Model file for the job. Use its own axes, mm. A direction names the side the tool comes from. Round coordinates to 2 decimals unless told otherwise and drop trailing zeros. Order: outer loops, then holes, each group sorted by start corner. A loop starts at its lowest first (then second) coordinate and runs counter-clockwise, first axis right, second up. Notation, with made-up numbers: (21, 48) - (29, 48) arc R29 ccw to (29, 76) - close; hole circle Ø9 at (62, 1.5). An arc over 180 degrees is marked (long way). Put each result on its own line as item: value. Start each with the question number.
Item 1: Mould opens along Y. For faces 5 (the face through (-33, 42.5, 49)), 6 (the face through (-33.45, -34.95, 14.95)), 7 (the face through (-37, 1, 49)) say: pulls with the +Y half, pulls with the -Y half, needs draft (parallel to the pull), parting line crosses it, or undercut.
Item 2: Which spindle directions (+Z, -Z, +X, -X, +Y, -Y) get a long thin tool onto all of the face, cutting with end or side? Do faces 1 (the face through (-7.378, 10.417, 3.549)), 2 (the face through (-15, -22.5, 49)), 3 (the face through (-30, 32, 49)), 4 (the face through (-20.274, 0.057, 54.151)). Say none if no direction does.
Item 3: Saw through at A-A on z = 38.1. List the corners of the cut face in (x, y) (3 decimals).
Item 4: Pin check, flat tips, straight feed: pin 1 Ø24 at (x, z) = (-10.5, 39) entering from +Y; pin 2 Ø8.5 at (y, z) = (32.5, 63.5) entering from +X; pin 3 Ø5 at (x, z) = (10.5, 28.5) entering from -Y; pin 4 Ø3 at (x, y) = (-7, -12.13) entering from -Z. Stop position of each tip, or through.
Item 5: Saw through at C-C on x = 14. List the corners of the cut face in (y, z), plus the area to 3 significant figures.
Item 6: Probe probe 1 along Z at (x, y) = (-34.75, 32.5) (3 decimals); probe 2 along Y at (x, z) = (-32, 63); probe 3 along Y at (x, z) = (-29.5, 17.5). List the from-to ranges inside material, lowest first.
Item 7: Saw through at D-D on y = 4. List the corners of the cut face in (x, z).
Item 8: Saw through at B-B on y = -32.5. List the corners of the cut face in (x, z) (3 decimals), plus the area to 3 significant figures.
```python
from build123d import *

# Parameters (mm, degrees)
F1_DEPTH = 100
F3_DEPTH = 93
F4_R     = 10.75
F4_R_2   = 1.75
F5_DEPTH = 7.001
F6_R     = 3.325
F7_DEPTH = 7.001


with BuildPart() as f1:
    # F0 (on Top) → F1 (new body)
    with BuildSketch(Plane.XY):
        with BuildLine():
            Line((-30, -22.5), (0, -22.5))
            ThreePointArc((0, -22.5), (22.5, 0), (0, 22.5))
            Line((0, 22.5), (-30, 22.5))
            Line((-30, 22.5), (-30, 42.5))
            Line((-30, 42.5), (-37, 42.5))
            Line((-37, 42.5), (-37, -42.5))
            Line((-37, -42.5), (-30, -42.5))
            Line((-30, -42.5), (-30, -22.5))
        make_face()
    extrude(amount=F1_DEPTH)

    # F2 (on face) → F3 (cut)
    with BuildSketch(Plane.XY.offset(100)):
        with BuildLine():
            ThreePointArc((10.9589791569, -13.9946918808), (15.9804017395, -7.7831475152), (17.775, 0))
            ThreePointArc((17.775, 0), (15.9804017395, 7.7831475152), (10.9589791569, 13.9946918808))
            ThreePointArc((10.9589791569, 13.9946918808), (7.6371976915, 13.2287125761), (6.6395155094, 16.4884037675))
            ThreePointArc((6.6395155094, 16.4884037675), (-8.8876758914, 15.3935), (-17.5991912799, 2.493810597))
            ThreePointArc((-17.5991912799, 2.493810597), (-15.9461312513, 1.7044761952), (-15.275, 0))
            ThreePointArc((-15.275, 0), (-15.9461312513, -1.7044761952), (-17.5991912799, -2.493810597))
            ThreePointArc((-17.5991912799, -2.493810597), (-8.8876758914, -15.3935), (6.6395155094, -16.4884037675))
            ThreePointArc((6.6395155094, -16.4884037675), (7.6371976915, -13.2287125761), (10.9589791569, -13.9946918808))
        make_face()
        with BuildLine():
            ThreePointArc((6.6395155094, 16.4884037675), (7.6371976915, 13.2287125761), (10.9589791569, 13.9946918808))
            ThreePointArc((10.9589791569, 13.9946918808), (8.8871482138, 15.3938046508), (6.6395155094, 16.4884037675))
        make_face()
        with BuildLine():
            ThreePointArc((6.6395155094, 16.4884037675), (8.8871482138, 15.3938046508), (10.9589791569, 13.9946918808))
            ThreePointArc((10.9589791569, 13.9946918808), (11.2777106327, 14.662223267), (11.3871482138, 15.3938046508))
            ThreePointArc((11.3871482138, 15.3938046508), (9.4488056891, 17.8298959628), (6.6395155094, 16.4884037675))
        make_face()
        with BuildLine():
            ThreePointArc((11.3871482138, -15.3938046508), (11.2777106327, -14.662223267), (10.9589791569, -13.9946918808))
            ThreePointArc((10.9589791569, -13.9946918808), (8.8871482138, -15.3938046508), (6.6395155094, -16.4884037675))
            ThreePointArc((6.6395155094, -16.4884037675), (9.4488056891, -17.8298959628), (11.3871482138, -15.3938046508))
        make_face()
        with BuildLine():
            ThreePointArc((6.6395155094, -16.4884037675), (8.8871482138, -15.3938046508), (10.9589791569, -13.9946918808))
            ThreePointArc((10.9589791569, -13.9946918808), (7.6371976915, -13.2287125761), (6.6395155094, -16.4884037675))
        make_face()
        with BuildLine():
            ThreePointArc((-15.275, 0), (-15.9461312513, 1.7044761952), (-17.5991912799, 2.493810597))
            ThreePointArc((-17.5991912799, 2.493810597), (-17.775, 0), (-17.5991912799, -2.493810597))
            ThreePointArc((-17.5991912799, -2.493810597), (-15.9461312513, -1.7044761952), (-15.275, 0))
        make_face()
        with BuildLine():
            ThreePointArc((-17.5991912799, -2.493810597), (-17.775, 0), (-17.5991912799, 2.493810597))
            ThreePointArc((-17.5991912799, 2.493810597), (-20.275, 0), (-17.5991912799, -2.493810597))
        make_face()
    extrude(amount=-F3_DEPTH, mode=Mode.SUBTRACT)

    # F4 (on face) → F5 (cut, through all)
    with BuildSketch(Plane.XY.offset(7)):
        Circle(F4_R)
        with Locations((14, 0)):
            Circle(F4_R_2)
        with Locations((-6.998768, 12.1250668651)):
            Circle(F4_R_2)
        with Locations((-6.998768, -12.1250668651)):
            Circle(F4_R_2)
    extrude(amount=-F5_DEPTH, mode=Mode.SUBTRACT)

    # F6 (on face) → F7 (cut, through all)
    with BuildSketch(Plane.YZ.offset(-30)):
        with Locations((32.5, 12.7)):
            Circle(F6_R)
        with Locations((-32.5, 12.7)):
            Circle(F6_R)
        with Locations((-32.5, 63.5)):
            Circle(F6_R)
        with Locations((32.5, 63.5)):
            Circle(F6_R)
        with Locations((-32.5, 38.1)):
            Circle(F6_R)
        with Locations((32.5, 38.1)):
            Circle(F6_R)
    extrude(amount=-F7_DEPTH, mode=Mode.SUBTRACT)


solid = f1.part
```
Results found:
1. face 5: pulls with the +Y half
1. face 6: undercut
1. face 7: needs draft
2. face 1: +Z, -Z
2. face 2: +Z, -Z, +X, -Y
2. face 3: +Z, -Z, +X, +Y
2. face 4: +Z
3. outline: (-37, -42.5) - (-30, -42.5) - (-30, -35.825) - (-37, -35.825) - close; (-37, -29.175) - (-30, -29.175) - (-30, -22.5) - (0, -22.5) arc R22.5 ccw to (0, 22.5) - (-30, 22.5) - (-30, 29.175) - (-37, 29.175) - close; (-37, 35.825) - (-30, 35.825) - (-30, 42.5) - (-37, 42.5) - close; hole (-17.599, -2.494) arc R17.775 ccw to (6.64, -16.488) arc R2.5 ccw (long way) to (10.959, -13.995) arc R17.775 ccw to (10.959, 13.995) arc R2.5 ccw (long way) to (6.64, 16.488) arc R17.775 ccw to (-17.599, 2.494) arc R2.5 ccw (long way) to start
4. pin 1: stops at y = 22.5
4. pin 2: stops at x = -30
4. pin 3: stops at y = -21.03
4. pin 4: passes through
5. outline: (-17.61, 0) - (-1.75, 0) - (-1.75, 7) - (-10.95, 7) - (-10.95, 100) - (-17.61, 100) - close; (1.75, 0) - (17.61, 0) - (17.61, 100) - (10.95, 100) - (10.95, 7) - (1.75, 7) - close
5. area: 1,460 mm²
6. probe 1: z = 0 to 9.375, 16.025 to 34.775, 41.425 to 60.175, 66.825 to 100
6. probe 2: y = -42.5 to -35.79, -29.21 to 29.21, 35.79 to 42.5
6. probe 3: y = -22.5 to 22.5
7. outline: (-37, 0) - (-9.98, 0) - (-9.98, 7) - (-17.32, 7) - (-17.32, 100) - (-37, 100) - close; (9.98, 0) - (22.14, 0) - (22.14, 100) - (17.32, 100) - (17.32, 7) - (9.98, 7) - close
8. outline: (-37, 0) - (-30, 0) - (-30, 9.375) - (-37, 9.375) - close; (-37, 16.025) - (-30, 16.025) - (-30, 34.775) - (-37, 34.775) - close; (-37, 41.425) - (-30, 41.425) - (-30, 60.175) - (-37, 60.175) - close; (-37, 66.825) - (-30, 66.825) - (-30, 100) - (-37, 100) - close
8. area: 560 mm²
